Here's how the part is built. I have some questions about the finished solid (model axes, mm). Coordinates: 2 decimals unless noted, no trailing zeros. Loops run counter-clockwise (first coordinate to the right, second up) from the corner with the lowest first, then second, coordinate; pieces in that order, holes last. Notation, with made-up numbers: (15.25, 59) -> (48.25, 59) arc R17 ccw to (48.25, 68) -> close; hole circle Ø9 at (35, 56.5). An arc over 180 degrees is marked (long way). Use CSV: the item, a comma, the result in double quotes. Start each with the question number.
from build123d import *

# Parameters (mm, degrees)
SKETCH_1_R      = 50
SKETCH_1_R_2    = 3
EXTRUDE_1_DEPTH = 20


with BuildPart() as part:
    # 草图1 → 凸台-拉伸1 (new body)
    with BuildSketch(Plane.XY):
        Circle(SKETCH_1_R)
        with Locations((-18, 0)):
            Circle(SKETCH_1_R_2, mode=Mode.SUBTRACT)
        with Locations((0, 18)):
            Circle(SKETCH_1_R_2, mode=Mode.SUBTRACT)
        with Locations((18, 0)):
            Circle(SKETCH_1_R_2, mode=Mode.SUBTRACT)
        with Locations((0, -18)):
            Circle(SKETCH_1_R_2, mode=Mode.SUBTRACT)
        with Locations((-35, 0)):
            Circle(SKETCH_1_R_2, mode=Mode.SUBTRACT)
        with Locations((-17.5, 30.310889132)):
            Circle(SKETCH_1_R_2, mode=Mode.SUBTRACT)
        with Locations((17.5, 30.310889132)):
            Circle(SKETCH_1_R_2, mode=Mode.SUBTRACT)
        with Locations((35, 0)):
            Circle(SKETCH_1_R_2, mode=Mode.SUBTRACT)
        with Locations((17.5, -30.310889132)):
            Circle(SKETCH_1_R_2, mode=Mode.SUBTRACT)
        with Locations((-17.5, -30.310889132)):
            Circle(SKETCH_1_R_2, mode=Mode.SUBTRACT)
    extrude(amount=EXTRUDE_1_DEPTH)


solid = part.part
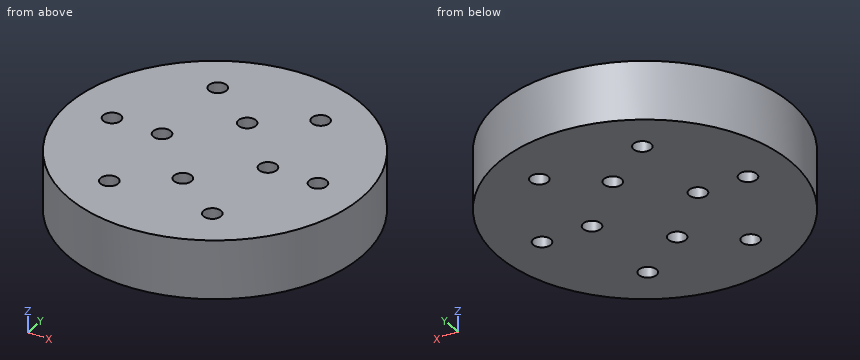
1) I want a section at B-B, the plane x = -18. Please give me the cut outline in (y, z).
2) I want a section at C-C, the plane y = 18. Please give me the cut outline in (x, z), plus the area to 3 significant figures.
3) Please list where these lines run through material, in increasing order: L1, parallel to Y at x = 0, z = 13.25; L2, parallel to Y at x = -17.5, z = 5; L3, parallel to Y at x = -1, z = 13.25. Write a range as [from, to].
4) I want a section at D-D, the plane z = 10.25. State how many separate pieces and enclosed holes the cut face has, plus the area to 3 significant figures.
5) I want a section at A-A, the plane x = 0. Please give me the cut outline in (y, z), plus the area to 3 significant figures.
6) For P1, Ø7, axis at x = 18, y = 0, coming from the -Z side; P2, Ø3.5, axis at x = 0, y = 18, coming from the -Z side; P3, Ø1.5, axis at y = -31.5, z = 17, coming from the -X side; P4, Ø1.5, axis at y = -24.5, z = 4.5, coming from the +X side, each with a flat end and sliding along its axis, tell me the tip position at first contact or that it passes through.
Return value:
1,outline,"(-46.65, 0) -> (-33.27, 0) -> (-33.27, 20) -> (-46.65, 20) -> close; (-27.35, 0) -> (-3, 0) -> (-3, 20) -> (-27.35, 20) -> close; (3, 0) -> (27.35, 0) -> (27.35, 20) -> (3, 20) -> close; (33.27, 0) -> (46.65, 0) -> (46.65, 20) -> (33.27, 20) -> close"
2,outline,"(-46.65, 0) -> (-3, 0) -> (-3, 20) -> (-46.65, 20) -> close; (3, 0) -> (46.65, 0) -> (46.65, 20) -> (3, 20) -> close"
2,area,"1,750 mm²"
3,L1,"y = [-50, -21], [-15, 15], [21, 50]"
3,L2,"y = [-46.84, -33.31], [-27.31, -2.96], [2.96, 27.31], [33.31, 46.84]"
3,L3,"y = [-49.99, -20.83], [-15.17, 15.17], [20.83, 49.99]"
4,separate pieces,"1"
4,enclosed holes,"10"
4,area,"7,570 mm²"
5,outline,"(-50, 0) -> (-21, 0) -> (-21, 20) -> (-50, 20) -> close; (-15, 0) -> (15, 0) -> (15, 20) -> (-15, 20) -> close; (21, 0) -> (50, 0) -> (50, 20) -> (21, 20) -> close"
5,area,"1,760 mm²"
6,P1,"stops at z = 0"
6,P2,"passes through"
6,P3,"stops at x = -39.43"
6,P4,"stops at x = 44"
